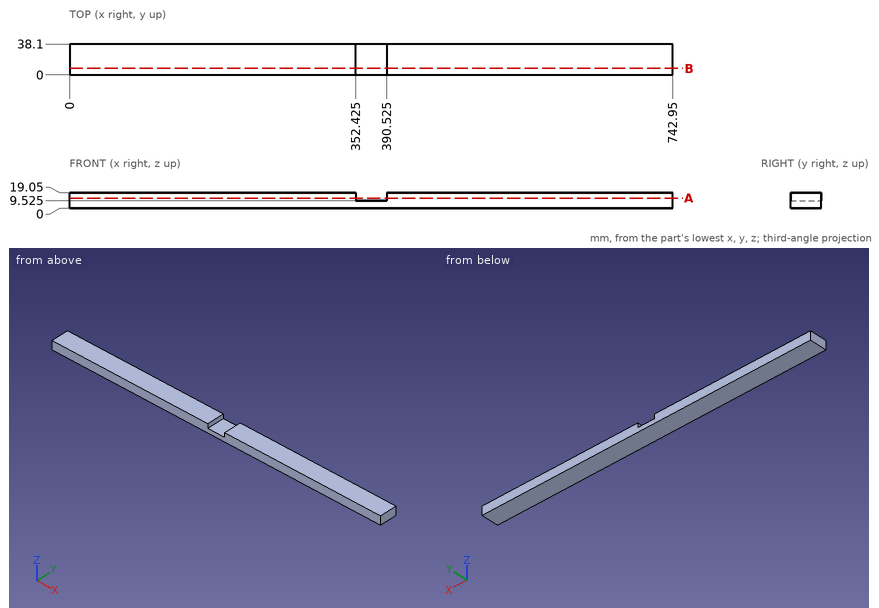
Here's the drawing with two shaded views (mm, measured from the low corner). I have some questions. Give positions to 0.01 mm unless a question says otherwise; leave off trailing zeros. Loops run counter-clockwise (first coordinate to the right, second up) from the corner with the lowest first, then second, coordinate; pieces in that order, holes last. Notation, with made-up numbers: M 81.5,-23 L 101.5,-23 A16 cw 101.5,-13 Z; hole C 28,60.5 d5. An arc over 180 degrees is marked long. Use one line per item in the form item = value. Start each with the question number.
(1) I want a section at A-A, the plane z = 12.75. Write out the boundary of the cut face in (x, y) (3 decimals).
(2) I want a section at B-B, the plane y = 8. Write out the boundary of the cut face in (x, z) (3 decimals).
(3) I'm going to push a flat-ended pin straight in: P1, Ø19, axis at x = 370.5, y = 19, coming from the +Z side (3 decimals). Where does the tip first touch, or does it pass through?
(4) Please list where these lines run through material, in increasing order: line 1 (X direction, y = 8, z = 13) (3 decimals); line 2 (Z direction, x = 368.5, y = 22.5) (3 decimals).
Worked out:
q1.outline = M 0,0 L 352.425,0 L 352.425,38.1 L 0,38.1 Z; M 390.525,0 L 742.95,0 L 742.95,38.1 L 390.525,38.1 Z
q2.outline = M 0,0 L 742.95,0 L 742.95,19.05 L 390.525,19.05 L 390.525,9.525 L 352.425,9.525 L 352.425,19.05 L 0,19.05 Z
q3.P1 = 9.525
q4.line_1 = 0 to 352.425, 390.525 to 742.95
q4.line_2 = 0 to 9.525
